Geometry check sheet. Reference: the model listing, model coordinates, mm. A direction names the side the tool comes from. Round coordinates to 2 decimals unless told otherwise and drop trailing zeros. Loops run counter-clockwise (first coordinate to the right, second up) from the corner with the lowest first, then second, coordinate; pieces in that order, holes last. Notation, with made-up numbers: (14, 89.25) - (18, 89.25) arc R17 cw to (18, 108.25) - close; hole circle Ø10 at (13, 49). An arc over 180 degrees is marked (long way). Write item = value, one per line.
```python
from build123d import *

# Parameters (mm, degrees)
SKETCH1_R               = 15
BOSS_EXTRUDE1_DEPTH     = 40
CUT_EXTRUDE1_DEPTH      = 40
CUT_EXTRUDE1_DEPTH_BACK = 40
SKETCH2_R               = 3.75
SKETCH4_R               = 1.5
CUT_EXTRUDE2_DEPTH      = 8
SKETCH5_R               = 2.5
CUT_EXTRUDE3_DEPTH      = 8
FILLET1_R               = 5
CHAMFER1_SIZE           = 2
FILLET2_R               = 2.5


with BuildPart() as part:
    # Sketch1 → Boss-Extrude1 (new body)
    with BuildSketch(Plane(origin=(0, 0, 0), x_dir=(1, 0, 0), z_dir=(0, 1, 0))):
        with Locations(Location((0, 0, 0), (0, 0, 270))):
            Circle(SKETCH1_R)
    extrude(amount=BOSS_EXTRUDE1_DEPTH)

    # Sketch2 → Cut-Extrude1 (cut, two sides: drawn at the far end of the back side and taken through both)
    with BuildSketch(Plane.XY.offset(-CUT_EXTRUDE1_DEPTH_BACK)):
        Polygon((10, 7.5), (0, 7.5), (-10, 7.5), (-10, 24.5), (10, 24.5), align=None)
        with Locations(Location((0, 33, 0), (0, 0, 89.999999996))):
            Circle(SKETCH2_R)
    extrude(amount=CUT_EXTRUDE1_DEPTH + CUT_EXTRUDE1_DEPTH_BACK, mode=Mode.SUBTRACT)

    # Sketch4 → Cut-Extrude2 (cut)
    with BuildSketch(Plane(origin=(0, 40, 0), x_dir=(1, 0, 0), z_dir=(0, 1, 0))):
        with Locations(Location((0, 0, 0), (0, 0, 270))):
            Circle(SKETCH4_R)
    extrude(amount=-CUT_EXTRUDE2_DEPTH, mode=Mode.SUBTRACT)

    # Sketch5 → Cut-Extrude3 (cut)
    with BuildSketch(Plane.XZ):
        with Locations(Location((0, 0, 0), (0, 0, 270))):
            Circle(SKETCH5_R)
    extrude(amount=-CUT_EXTRUDE3_DEPTH, mode=Mode.SUBTRACT)

    # Fillet1
    # the kernel refuses this fillet: 5 mm, written as the material it takes off along each edge
    with BuildSketch(Plane(origin=(0, 40, 0), x_dir=(0, 0, 1), z_dir=(-1, 0, 0))) as fillet1_piece_1:
        with BuildLine():
            CenterArc((15 - FILLET1_R, -FILLET1_R), FILLET1_R, 0, 90)
            Line((15 - FILLET1_R, 0), (15, 0))
            Line((15, 0), (15, -FILLET1_R))
        make_face()
    revolve(axis=Axis((0, 40, 0), (0, 1, 0)), mode=Mode.SUBTRACT)

    # Chamfer1
    chamfer1_edges = [part.edges().sort_by_distance(p)[0] for p in [
        (0, 40, -1.5),
    ]]
    chamfer(chamfer1_edges, length=CHAMFER1_SIZE)

    # Fillet2
    fillet2_edges = [part.edges().sort_by_distance(p)[0] for p in [
        (0, 0, -15),
    ]]
    fillet(fillet2_edges, radius=FILLET2_R)


solid = part.part
```
(1) Section check A-A (z = -12). State how many separate pieces and enclosed holes the cut face has, then the cut area to 3 significant figures.
Answers follow:
separate_pieces = 2
enclosed_holes = 1
area = 342 mm²
(2) Scan lines: L1, parallel to Y at x = -5.5, z = -2.5; L2, parallel to X at y = 3, z = 0; L3, parallel to Y at x = -3, z = -3. Record each from-to range of solid material in increasing order. Write a range as [from, to].
Answers follow:
L1 = [0, 7.5], [24.5, 40]
L2 = [-15, -2.5], [2.5, 15]
L3 = [0, 7.5], [24.5, 30.75], [35.25, 40]
(3) Section check D-D (z = 0). Enter the section's corners in (x, y).
Answers follow:
outline = (-15, 2.5) arc R2.5 ccw to (-12.5, 0) - (-2.5, 0) - (-2.5, 7.5) - (-10, 7.5) - (-10, 24.5) - (10, 24.5) - (10, 7.5) - (2.5, 7.5) - (2.5, 0) - (12.5, 0) arc R2.5 ccw to (15, 2.5) - (15, 35) arc R5 ccw to (10, 40) - (3.5, 40) - (1.5, 38) - (1.5, 36.44) arc R3.75 cw (long way) to (-1.5, 36.44) - (-1.5, 38) - (-3.5, 40) - (-10, 40) arc R5 ccw to (-15, 35) - close
(4) Set-up check for faces 1 (the flat face through (-10, 16, 0)), 2 (the cylindrical face through (12.65, 18.52, 8.06)), 3 (the cylindrical face through (-0.575, 37.229, 1.386)): record each of +Z, -Z, +X, -X, +Y, -Y from which the full face is reachable in a straight line by a thin tool's end or side.
Answers follow:
face_1 = +Z, -Z
face_2 = +Y, -Y
face_3 = +Y
(5) Section check C-C (x = 0). Enter the section's corners in (y, z), then the cut area to 3 significant figures.
Answers follow:
outline = (0, -12.5) arc R2.5 ccw to (2.5, -15) - (7.5, -15) - (7.5, -2.5) - (0, -2.5) - close; (0, 2.5) - (7.5, 2.5) - (7.5, 15) - (2.5, 15) arc R2.5 ccw to (0, 12.5) - close; (24.5, -15) - (29.25, -15) - (29.25, 15) - (24.5, 15) - close; (36.75, -14.68) arc R5 ccw to (40, -10) - (40, -3.5) - (38, -1.5) - (36.75, -1.5) - close; (36.75, 1.5) - (38, 1.5) - (40, 3.5) - (40, 10) arc R5 ccw to (36.75, 14.68) - close
area = 401 mm²
(6) Gauge pin test, flat ends, axial feed: pin 1 (1.5 mm diameter, centred on y = 17.5, z = 8.5, fed in from -X); pin 2 (4.5 mm diameter, centred on x = 0, z = 0, fed in from +Y); pin 3 (3.5 mm diameter, centred on x = 0, z = 0, fed in from -Y); pin 4 (4.5 mm diameter, centred on x = 0, y = 33, fed in from +Z). Record the tip position at first contact, or that the pin passes through.
Answers follow:
pin_1 = -12.84
pin_2 = 38.75
pin_3 = 24.5
pin_4 = through
(7) Mould release check, pull along Y, two halves, no side actions. Record for faces 4 (the conical face through (0.488, 38.125, 1.55)), 5 (the flat face through (0, 24.5, 0)), 6 (the cylindrical face through (-2.44, 3.7, 0.54)): pulls with the +Y half, pulls with the -Y half, needs draft (parallel to the pull), parting line crosses it, or undercut.
Answers follow:
face_4 = pulls with the +Y half
face_5 = undercut
face_6 = needs draft
(8) Section check B-B (y = 16). Enter the section's corners in (x, z), then the cut area to 3 significant figures.
Answers follow:
outline = (-10, -11.18) - (-10, 11.18) arc R15 ccw to start; (10, -11.18) arc R15 ccw to (10, 11.18) - close
area = 155 mm²
